from build123d import *

# Parameters (mm, degrees)
SKETCH1_R           = 6
BOSS_EXTRUDE1_DEPTH = 5
SKETCH2_R           = 2.5
CUT_EXTRUDE1_DEPTH  = 2
SKETCH3_R           = 1
CUT_EXTRUDE2_DEPTH  = 2
FILLET1_R           = 1


with BuildPart() as part:
    # Sketch1 → Boss-Extrude1 (new body)
    with BuildSketch(Plane(origin=(0, 0, 0), x_dir=(1, 0, 0), z_dir=(0, 1, 0))):
        Circle(SKETCH1_R)
    extrude(amount=BOSS_EXTRUDE1_DEPTH)

    # Sketch2 → Cut-Extrude1 (cut)
    with BuildSketch(Plane(origin=(0, 5, 0), x_dir=(1, 0, 0), z_dir=(0, 1, 0))):
        Circle(SKETCH2_R)
    extrude(amount=-CUT_EXTRUDE1_DEPTH, mode=Mode.SUBTRACT)

    # Sketch3 → Cut-Extrude2 (cut)
    with BuildSketch(Plane.XZ):
        Circle(SKETCH3_R)
    extrude(amount=-CUT_EXTRUDE2_DEPTH, mode=Mode.SUBTRACT)

    # Fillet1
    fillet1_edges = [part.edges().sort_by_distance(p)[0] for p in [
        (-1, 2, 0),
    ]]
    fillet(fillet1_edges, radius=FILLET1_R)


solid = part.part
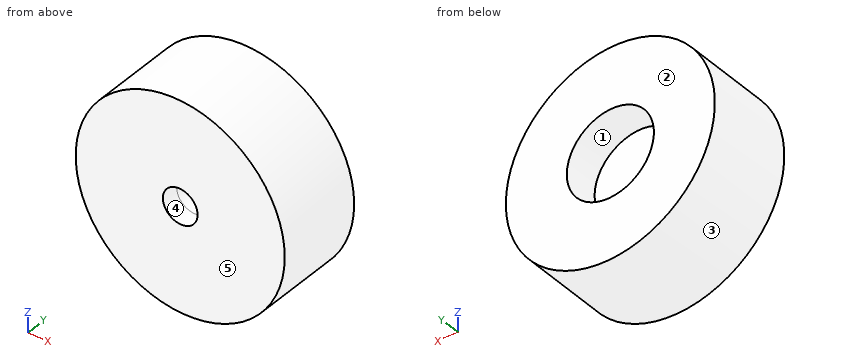
Verification items for the finished model (mm, model axes). Face numbers are marked on the shaded views. A direction names the side the tool comes from. Give positions to 0.01 mm unless a question says otherwise; leave off trailing zeros. Write each loop counter-clockwise with the first axis right and the second up, starting at its lowest first coordinate (ties: lowest second). Pieces come first, ordered by that corner, then holes.
(1) Material ranges on line 1 (Z direction, x = 0, y = 3.95); line 2 (Z direction, x = 0, y = 0.4), recorded low to high.
(2) Cross-section at B-B (y = 4). Enter the section's corners in (x, z).
(3) Cross-section at D-D (y = 2.8). Enter the section's corners in (x, z), plus the area to 3 significant figures.
(4) Cross-section at C-C (z = 0). Enter the section's corners in (x, y).
(5) Access from +Z, -Z, +X, -X, +Y, -Y to the whole of each face (thin tool, end or side, straight path). Record for the marked faces 1 and 2.
(6) Mould release check, pull along Z, two halves, no side actions. Record for the marked faces 3, 4 and 5: +Z half, -Z half, draft (parallel to the pull), parting line (faces both ways), or undercut.
(7) Gauge pin test, flat ends, axial feed: pin 1 (1 mm diameter, centred on y = 0.5, z = 5, fed in from +X); pin 2 (3 mm diameter, centred on x = 3, y = 3, fed in from +Z); pin 3 (1.5 mm diameter, centred on y = 4, z = -1.5, fed in from +X). Record the tip position at first contact, or that the pin passes through.
(8) Cross-section at A-A (x = 0). Enter the section's corners in (y, z), plus the area to 3 significant figures.
Worked out:
1. line 1: z = -6 to -2.5, 2.5 to 6
1. line 2: z = -6 to -1, 1 to 6
2. outline: circle Ø12 at (0, 0); hole circle Ø5 at (0, 0)
3. outline: circle Ø12 at (0, 0)
3. area: 113 mm2
4. outline: (-6, 0) - (-1, 0) - (-1, 1) arc R1 cw to (1, 1) - (1, 0) - (6, 0) - (6, 5) - (2.5, 5) - (2.5, 3) - (-2.5, 3) - (-2.5, 5) - (-6, 5) - close
5. face 1: +Y
5. face 2: +Z, -Z, +X, -X, +Y
6. face 3: parting line
6. face 4: undercut
6. face 5: draft
7. pin 1: stops at x = 3.97
7. pin 2: stops at z = 5.81
7. pin 3: stops at x = 5.95
8. outline: (0, -6) - (5, -6) - (5, -2.5) - (3, -2.5) - (3, 2.5) - (5, 2.5) - (5, 6) - (0, 6) - (0, 1) - (1, 1) arc R1 cw to (1, -1) - (0, -1) - close
8. area: 46.4 mm2
